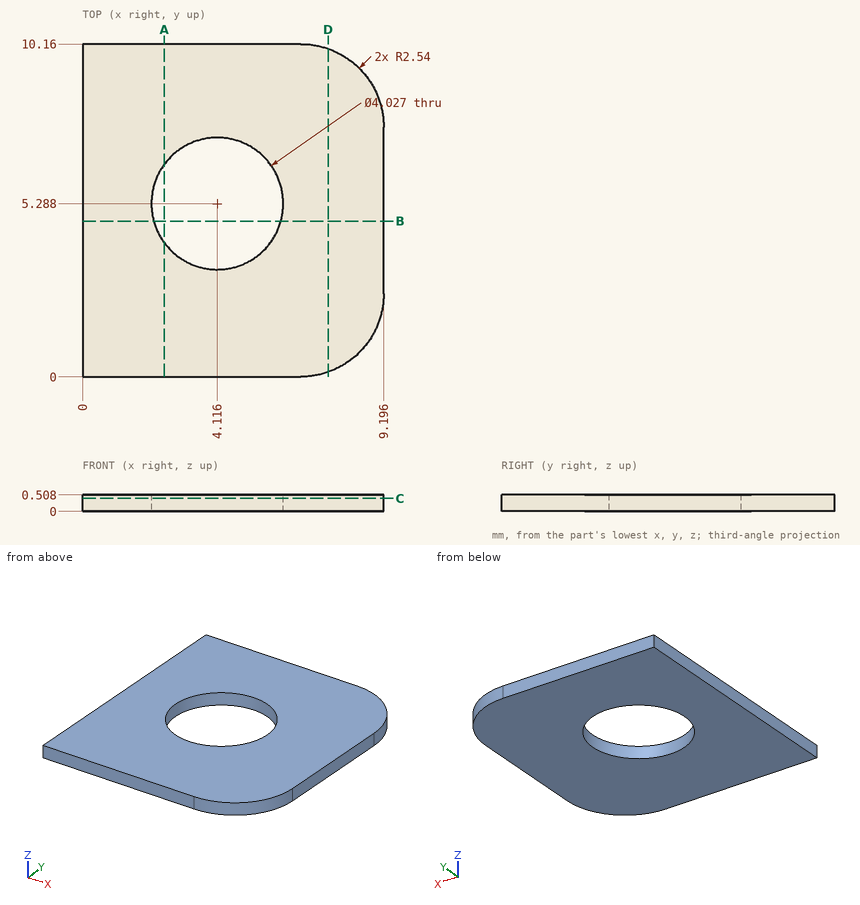
Study the drawing (mm; zero at the part's minimum x, y, z) and answer. Give positions to 0.01 mm unless a question says otherwise; leave off trailing zeros. Write each loop counter-clockwise with the first axis right and the second up, starting at its lowest first coordinate (ties: lowest second). Pieces come first, ordered by that corner, then holes. Notation, with made-up numbers: (-19.5, 0.5) - (26.5, 0.5) arc R32 cw to (26.5, 30.5) - close; hole circle Ø1 at (7, -38). An arc over 180 degrees is marked (long way). One line per question, with ' | ' between items. Start each with the question number.
1. Section A-A, the plane x = 2.5 is taken. Determine the outline of the cut face in (y, z).
2. Section D-D, the plane x = 7.5 is taken. Determine the outline of the cut face in (y, z) (1 decimal).
3. Straight lines are drawn through the part: line 1 (Y direction, x = 3.25, z = 0.3) (1 decimal); line 2 (X direction, y = 5, z = 0.25); line 3 (X direction, y = 4.75, z = 0.1) (1 decimal). For each, find the intervals that lie inside material, in ascending order.
4. Given P1, Ø1.5, axis at x = 5.5, y = 4.5, coming from the -Z side, flat-ended and moving along its own axis, determine where the tip first touches the part or whether it passes through.
5. Section C-C, the plane z = 0.4 is taken. Determine the outline of the cut face in (x, y).
6. Section B-B, the plane y = 4.75 is taken. Determine the outline of the cut face in (x, z) (1 decimal).
Result:
1) outline: (0, 0) - (4.09, 0) - (4.09, 0.51) - (0, 0.51) - close; (6.49, 0) - (10.16, 0) - (10.16, 0.51) - (6.49, 0.51) - close
2) outline: (0.1, 0) - (10, 0) - (10, 0.5) - (0.1, 0.5) - close
3) line 1: y = 0 to 3.5, 7.1 to 10.2 | line 2: x = 0 to 2.12, 6.11 to 9.2 | line 3: x = 0 to 2.2, 6.1 to 9.2
4) P1: stops at z = 0
5) outline: (0, 0) - (6.66, 0) arc R2.54 ccw to (9.2, 2.54) - (9.2, 7.62) arc R2.54 ccw to (6.66, 10.16) - (0, 10.16) - close; hole circle Ø4.03 at (4.12, 5.29)
6) outline: (0, 0) - (2.2, 0) - (2.2, 0.5) - (0, 0.5) - close; (6.1, 0) - (9.2, 0) - (9.2, 0.5) - (6.1, 0.5) - close
